Could you check a few things on this model? Use its own coordinates, in mm. A direction names the side the tool comes from. Round coordinates to 2 decimals unless told otherwise and drop trailing zeros. Order: outer loops, then holes, each group sorted by start corner. A loop starts at its lowest first (then second) coordinate and runs counter-clockwise, first axis right, second up.
Autodesk Inventor part; units mm, degrees
ref_plane "Plano de trabajo1" through (-28.0665, -74.268, 27.7) normal (0, 0, -1) x (0, 1, 0)
ref_plane "YZ Plane" through (0, 0, 0) normal (1, 0, 0) x (0, 1, 0)
ref_plane "XZ Plane" through (0, 0, 0) normal (0, 1, 0) x (-1, 0, 0)
sketch "Boceto1" plane through (0, 0, 0) normal (0, 0, 1) x (1, 0, 0)
  line L0 (-20.0665, -74.268) -> (20.3335, -74.268)
  line L1 (-20.0665, -54.068) -> (-20.0665, -74.268)
  line L2 (20.3335, -74.268) -> (20.3335, -54.068)
  circle A0 centre (24.7835, -69.268) radius 2.2
  circle A1 centre (24.7835, -59.068) radius 2.2
  line L3 (20.3335, -54.068) -> (20.3335, -74.268)
  line L4 (20.3335, -54.068) -> (28.3335, -54.068)
  line L5 (28.3335, -54.068) -> (28.3335, -74.268)
  line L6 (20.3335, -74.268) -> (28.3335, -74.268)
  line L7 (-20.0665, -74.268) -> (-28.0665, -74.268)
  circle A2 centre (-24.5165, -69.268) radius 2.2
  circle A3 centre (-24.5165, -59.068) radius 2.2
  line L8 (-20.0665, -54.068) -> (-20.0665, -74.268)
  line L9 (-20.0665, -54.068) -> (-28.0665, -54.068)
  line L10 (-28.0665, -74.268) -> (-28.0665, -54.068)
  line L11 (-20.0665, -74.268) -> (-28.0665, -74.268)
  line L12 (-20.0665, -66.768) -> (-25.0665, -66.768)
  line L13 (-25.0665, -61.568) -> (-25.0665, -66.768)
  line L14 (-20.0665, -61.568) -> (-25.0665, -61.568)
  line L15 (-20.0665, -54.068) -> (-20.0665, -74.268)
  line L16 (20.3335, -54.068) -> (-20.0665, -54.068)
  line L17 (20.3335, -74.268) -> (20.3335, -54.068)
  line L18 (-20.0665, -74.268) -> (20.3335, -74.268)
  circle A4 centre (-10.3665, -64.168) radius 3.1
  line L19 (-28.0665, -74.268) -> (-28.0665, -77.268)
  line L20 (-28.0665, -77.268) -> (-31.0665, -77.268)
  line L21 (28.3335, -54.068) -> (31.3335, -54.068)
  line L22 (31.3335, -54.068) -> (31.3335, -51.068)
  line L23 (31.3335, -51.068) -> (28.3335, -51.068)
  line L24 (28.3335, -51.068) -> (28.3335, -54.068)
  line L25 (31.3335, -51.068) -> (-31.0665, -51.068)
  line L26 (-31.0665, -51.068) -> (-31.0665, -77.268)
  line L27 (-31.0665, -77.268) -> (31.3335, -77.268)
  line L28 (31.3335, -77.268) -> (31.3335, -51.068)
  line L29 (-31.0665, -51.068) -> (-23.0665, -51.068)
  line L30 (-23.0665, -51.068) -> (-23.0665, -43.068)
  line L31 (-23.0665, -43.068) -> (-31.0665, -43.068)
  line L32 (-31.0665, -43.068) -> (-31.0665, -51.068)
  line L33 (-31.0665, -77.268) -> (-23.0665, -77.268)
  line L34 (-23.0665, -77.268) -> (-23.0665, -85.268)
  line L35 (-23.0665, -85.268) -> (-31.0665, -85.268)
  line L36 (-31.0665, -85.268) -> (-31.0665, -77.268)
  line L37 (31.3335, -77.268) -> (23.3335, -77.268)
  line L38 (23.3335, -77.268) -> (23.3335, -85.268)
  line L39 (23.3335, -85.268) -> (31.3335, -85.268)
  line L40 (31.3335, -85.268) -> (31.3335, -77.268)
  line L41 (31.3335, -51.068) -> (23.3335, -51.068)
  line L42 (23.3335, -51.068) -> (23.3335, -43.068)
  line L43 (23.3335, -43.068) -> (31.3335, -43.068)
  line L44 (31.3335, -43.068) -> (31.3335, -51.068)
  line L45 (-27.0665, -43.068) -> (-27.0665, -47.068)
  circle A5 centre (-27.0665, -47.068) radius 2.1
  line L46 (-27.0665, -85.268) -> (-27.0665, -81.268)
  circle A6 centre (-27.0665, -81.268) radius 2.1
  line L47 (27.3335, -43.068) -> (27.3335, -47.068)
  circle A7 centre (27.3335, -47.068) radius 2.1
  line L48 (27.3335, -85.268) -> (27.3335, -81.268)
  circle A8 centre (27.3335, -81.268) radius 2.1
  line L49 (-28.0665, -54.068) -> (28.3335, -54.068)
  line L50 (28.3335, -54.068) -> (28.3335, -74.268)
  line L51 (28.3335, -74.268) -> (-28.0665, -74.268)
  line L52 (-28.0665, -74.268) -> (-28.0665, -54.068)
  line L53 (28.5835, -53.818) -> (-28.3165, -53.818)
  line L54 (-28.3165, -53.818) -> (-28.3165, -74.518)
  line L55 (-28.3165, -74.518) -> (28.5835, -74.518)
  line L56 (28.5835, -74.518) -> (28.5835, -53.818)
  line L57 (-20.3165, -53.818) -> (-20.3165, -74.518)
  line L58 (20.5835, -74.518) -> (20.5835, -53.818)
  line L59 (-25.0665, -61.568) -> (-20.0665, -66.768)
  line L60 (-19.0665, -69.168) -> (-26.0665, -69.168)
  line L61 (-26.0665, -69.168) -> (-26.0665, -59.168)
  line L62 (-26.0665, -59.168) -> (-19.0665, -59.168)
  line L63 (-19.0665, -59.168) -> (-19.0665, -69.168)
  line L64 (-19.0665, -69.168) -> (-26.0665, -59.168) construction
  line L65 (-26.0665, -69.168) -> (-19.0665, -59.168) construction
  point P0 (0, 0)
  point P1 (28.5835, -54.068)
  point P2 (28.3335, -53.818)
  point P3 (-20.3165, -61.568)
  point P4 (-20.3165, -66.768)
  point P5 (-22.5665, -64.168)
  point P6 (-20.3165, -69.168)
  point P7 (-20.3165, -59.168)
  dimension "d0" = 3
  dimension "d1" = 3
  dimension "d2" = 3
  dimension "d3" = 3
  dimension "d4" = 8
  dimension "d5" = 8
  dimension "d6" = 8
  dimension "d7" = 8
  dimension "d8" = 8
  dimension "d9" = 8
  dimension "d10" = 8
  dimension "d11" = 8
  dimension "d12" = 4
  dimension "d13" = 4.2
  dimension "d14" = 4
  dimension "d15" = 4.2
  dimension "d16" = 4
  dimension "d17" = 4.2
  dimension "d18" = 4
  dimension "d19" = 4.2
  dimension "d20" = 0.25
  dimension "d28" = 0.25
  dimension "d29" = 0.25
  dimension "d30" = 7
  dimension "d31" = 10
extrude "Extrusión1" add sketch "Boceto1" along normal blind 8 contours L57 L55 L19 L7 | L7 L10 L9 L57 L62 A3 L61 A2 L60 | L58 L4 L5 L6 | L6 L5 L21 L56 L55 L58 | L19 L55 L54 L53 L57 L9 L10 | L55 L56 L21 L28 L27 L19 | L58 L53 L24 L4 | A2 L61 L60 | L19 L20 L26 L25 L24 L53 L54 L55 | L24 L53 L56 L21 | L27 L34 L35 L36 L20 | L56 L53 L24 L23 L22 L21 | A3 L62 L61 | L25 L42 L43 L44 L23 | L32 L31 L30 L25 | L27 L40 L39 L38 | A0 | A1 picked at (-23.5885, -69.413) picked at (-23.5885, -58.923)
sketch "Boceto2" plane through (0, 0, 8) normal (0, 0, 1) x (1, 0, 0)
  line L0 (-23.0665, -85.268) -> (-23.0665, -77.268)
  line L1 (-23.0665, -77.268) -> (23.3335, -77.268)
  line L2 (23.3335, -77.268) -> (23.3335, -85.268)
  line L3 (23.3335, -85.268) -> (31.3335, -85.268)
  line L4 (31.3335, -85.268) -> (31.3335, -43.068)
  line L5 (31.3335, -43.068) -> (23.3335, -43.068)
  line L6 (23.3335, -43.068) -> (23.3335, -51.068)
  line L7 (23.3335, -51.068) -> (-23.0665, -51.068)
  line L8 (-23.0665, -51.068) -> (-23.0665, -43.068)
  line L9 (-23.0665, -43.068) -> (-31.0665, -43.068)
  line L10 (-31.0665, -43.068) -> (-31.0665, -85.268)
  line L11 (-31.0665, -85.268) -> (-23.0665, -85.268)
  circle A0 centre (-27.0665, -81.268) radius 2.1
  line L12 (20.5835, -74.518) -> (-20.3165, -74.518)
  line L13 (-20.3165, -53.818) -> (20.5835, -53.818)
  circle A1 centre (27.3335, -81.268) radius 2.1
  circle A2 centre (-27.0665, -47.068) radius 2.1
  circle A3 centre (27.3335, -47.068) radius 2.1
  line L14 (-23.0665, -85.268) -> (-23.0665, -77.268)
  line L15 (-23.0665, -77.268) -> (-31.0665, -77.268)
  line L16 (-23.0665, -77.268) -> (-15.0665, -77.268) construction
  line L17 (23.3335, -51.068) -> (31.3335, -51.068)
  line L18 (31.3335, -85.268) -> (31.3335, -43.068)
  line L19 (23.3335, -51.068) -> (31.3335, -51.068) construction
  line L20 (-31.0665, -77.268) -> (31.3335, -77.268)
  line L21 (31.3335, -77.268) -> (31.3335, -51.068)
  line L22 (31.3335, -51.068) -> (-31.0665, -51.068)
  line L23 (-31.0665, -51.068) -> (-31.0665, -77.268)
  line L24 (20.5835, -53.818) -> (20.5835, -74.518)
  line L25 (-20.3165, -74.518) -> (-20.3165, -69.168)
  line L26 (-20.3165, -59.168) -> (-20.3165, -53.818)
  line L27 (-20.3165, -69.168) -> (-26.0665, -69.168)
  line L28 (-26.0665, -69.168) -> (-26.0665, -59.168)
  line L29 (-26.0665, -59.168) -> (-20.3165, -59.168)
  line L30 (-20.3165, -59.168) -> (-20.3165, -69.168)
  point P0 (0, 0)
  dimension "d23" = 180
  dimension "d24" = 8
  dimension "d25" = 0
ref_plane "Plano de trabajo1" through (-28.0665, -74.268, 27.7) normal (0, 0, -1) x (0, 1, 0)
extrude "Extrusión2" add sketch "Boceto2" along normal up to surface (19.7 mm away) contours L15 L10 L22 L7 L17 L4 L20 L1 | L27 L28 L29 L30
sketch "Boceto3" plane through (-31.0665, -85.268, 0) normal (-1, 0, 0) x (0, 0, 1)
  line L0 (8, 16.1) -> (8, 26.1)
  line L1 (0, 26.1) -> (8, 26.1)
  line L2 (0, 26.1) -> (8, 26.1)
  line L3 (8, 26.1) -> (8, 16.1)
  line L4 (8, 16.1) -> (0, 16.1)
  line L5 (0, 16.1) -> (0, 26.1)
  point P0 (0, 85.268)
extrude "Extrusión3" cut sketch "Boceto3" against normal blind 8
sketch "Boceto4" plane through (-31.0665, -51.068, 27.7) normal (0, 0, 1) x (1, 0, 0)
  circle A0 centre (6.55, -18.2) radius 2.2
  circle A1 centre (6.55, -8) radius 2.2
  line L0 (11, -3) -> (11, -23.2)
  line L1 (11, -3) -> (3, -3)
  line L2 (3, -23.2) -> (3, -3)
  line L3 (11, -23.2) -> (3, -23.2)
  circle A2 centre (55.85, -18.2) radius 2.2
  circle A3 centre (55.85, -8) radius 2.2
  line L4 (51.4, -23.2) -> (51.4, -3)
  line L5 (51.4, -23.2) -> (59.4, -23.2)
  line L6 (59.4, -23.2) -> (59.4, -3)
  line L7 (51.4, -3) -> (59.4, -3)
  point P0 (31.0665, 51.068)
hole "Agujero1" at (-24.5165, -69.268, 27.7) at (-24.5165, -59.068, 27.7) at (24.7835, -69.268, 27.7) at (24.7835, -59.068, 27.7) direction (0, 0, -1) diameter 5.6 depth 15
fillet "Empalme1" radius 8 4 edges at (-23.0665, -77.268, 4) (23.3335, -77.268, 4) (-23.0665, -51.068, 4) (23.3335, -51.068, 4)
fillet "Empalme2" radius 2 4 edges at (-19.0668, -77.268, 8) (19.3337, -77.268, 8) (19.3337, -51.068, 8) (-19.0668, -51.068, 8)
equation "\"Radio_pliegue\" = Grosor"
equation "\"Anchura_desahogo_plegado\" = Grosor"
equation "\"Profundidad_desahogo_plegado\" = 0.5 * Grosor"
equation "\"Tamaño_destalonado\" = 4 * Grosor"
equation "\"Remanente_mínimo\" = 2 * Grosor"
equation "\"Radiodetransición\" = Radio_pliegue"
equation "\"Tamaño_de_radio_de_Jacobi\" = Radio_pliegue"
equation "\"TamañoSeparación\" = Grosor"
properties part number "Soporte_Servo"
Q1. For P1, Ø2, axis at x = -10, z = 16, coming from the +Y side; P2, Ø5, axis at x = 27.5, y = -82, coming from the +Z side; P3, Ø14, axis at x = -1, z = 9.5, coming from the -Y side, each with a flat end and sliding along its axis, tell me the tip position at first contact or that it passes through.
Q2. We'd pull the mould along Y, two halves only. Please class faces 1 (the flat face through (-27, -85.268, 4)), 2 (the flat face through (0, -74.518, 14)), 3 (the cylindrical face through (-27.34, -49.15, 3.94)), 4 (the flat face through (31.334, -64, 11)): released by +Y, released by -Y, zero draft, split by the parting line, or undercut.
Q3. Imagine slicing it at C-C, the plane z = 11.5. Please give me the cut outline in (x, y).
Q4. I need wall thicknesses on L1, parallel to Y at x = 20, z = 20.5; L2, parallel to X at y = -72.5, z = 11.25; L3, parallel to Y at x = -25, z = 26.5. Which ranges of each line are inside material? Lowest first, please.
Q5. Imagine slicing it at A-A, the plane x = 7.5. Please give me the cut outline in (y, z), then the cut area to 3 significant figures.
Q6. Imagine slicing it at B-B, the plane y = -54.5. Please give me the cut outline in (x, z).
Q7. For faces 5 (the cylindrical face through (-20.79, -48.66, 3.96)), 6 (the flat face through (26, -45, 8)), 7 (the flat face through (20.584, -64, 14)), 8 (the flat face through (-26, -59.168, 4)), 9 (the cylindrical face through (23.94, -61.74, 20.1)), which set-ups out of +Z, -Z, +X, -X, +Y, -Y let a thin tool reach every point of the face, with its end or its side?
Q8. Imagine slicing it at D-D, the plane z = 3. State how many separate pieces and enclosed holes the cut face has, then the cut area to 3 significant figures.
Filled in:
1. P1: stops at y = -51.07
1. P2: stops at z = 8
1. P3: stops at y = -77.27
2. face 1: released by -Y
2. face 2: undercut
2. face 3: undercut
2. face 4: zero draft
3. outline: (-31.07, -77.27) - (31.33, -77.27) - (31.33, -51.07) - (-31.07, -51.07) - close; hole (-20.32, -74.52) - (20.58, -74.52) - (20.58, -53.82) - (-20.32, -53.82) - close
4. L1: y = -77.27 to -74.52, -53.82 to -51.07
4. L2: x = -31.07 to -20.32, 20.58 to 31.33
4. L3: y = -77.27 to -72.03, -66.51 to -61.83, -56.31 to -51.07
5. outline: (-77.27, 0) - (-74.52, 0) - (-74.52, 27.7) - (-77.27, 27.7) - close; (-53.82, 0) - (-51.07, 0) - (-51.07, 27.7) - (-53.82, 27.7) - close
5. area: 152 mm2
6. outline: (-31.07, 0) - (-20.32, 0) - (-20.32, 27.7) - (-31.07, 27.7) - close; (20.58, 0) - (31.33, 0) - (31.33, 27.7) - (20.58, 27.7) - close
7. face 5: +Z, -Z, +Y
7. face 6: +Z, +X, -X, +Y
7. face 7: +Z, -Z
7. face 8: -Z, -X
7. face 9: +Z
8. separate pieces: 1
8. enclosed holes: 4
8. area: 936 mm2
